Input: dimensioned drawing with shaded views. Units: mm. Origin: part minimum x, y, z. Coordinates: 2 decimals unless noted, no trailing zeros. Order: outer loops, then holes, each group sorted by start corner. A loop starts at its lowest first (then second) coordinate and runs counter-clockwise, first axis right, second up. Notation, with made-up numbers: (24, 1.5) - (74, 1.5) arc R13 ccw to (74, 6.5) - close; hole circle Ø9 at (6, 77). An arc over 180 degrees is marked (long way). Answer as CSV lines item,"result". Start each with the question number.
Item 1: Section D-D (x = 203.2). Output: boundary loops of the cut face in (y, z) (1 decimal).
Item 2: Section A-A (x = 164.5). Output: boundary loops of the cut face in (y, z) (1 decimal).
Item 3: Section C-C (y = 2.7). State how many separate pieces and enclosed holes the cut face has, and give its area (3 significant figures).
Item 4: First-contact query: pin 1 (3.5 mm diameter, centred on x = 12.7, z = 124.36, fed in from +Y); pin 2 (7.5 mm diameter, centred on x = 237.74, z = 124.36, fed in from +Y). Flat tips, straight axial feed; report the tip coordinate or a pass-through.
Item 5: Section B-B (z = 67.31). Output: boundary loops of the cut face in (x, y) (1 decimal).
Item 6: Material intervals for line 1 along X through (y, z) = (2.15, 124) (1 decimal); line 2 along Z through (x, y) = (165, 4.55) (1 decimal); line 3 along X through (y, z) = (2.3, 65) (1 decimal), sorted ascending.
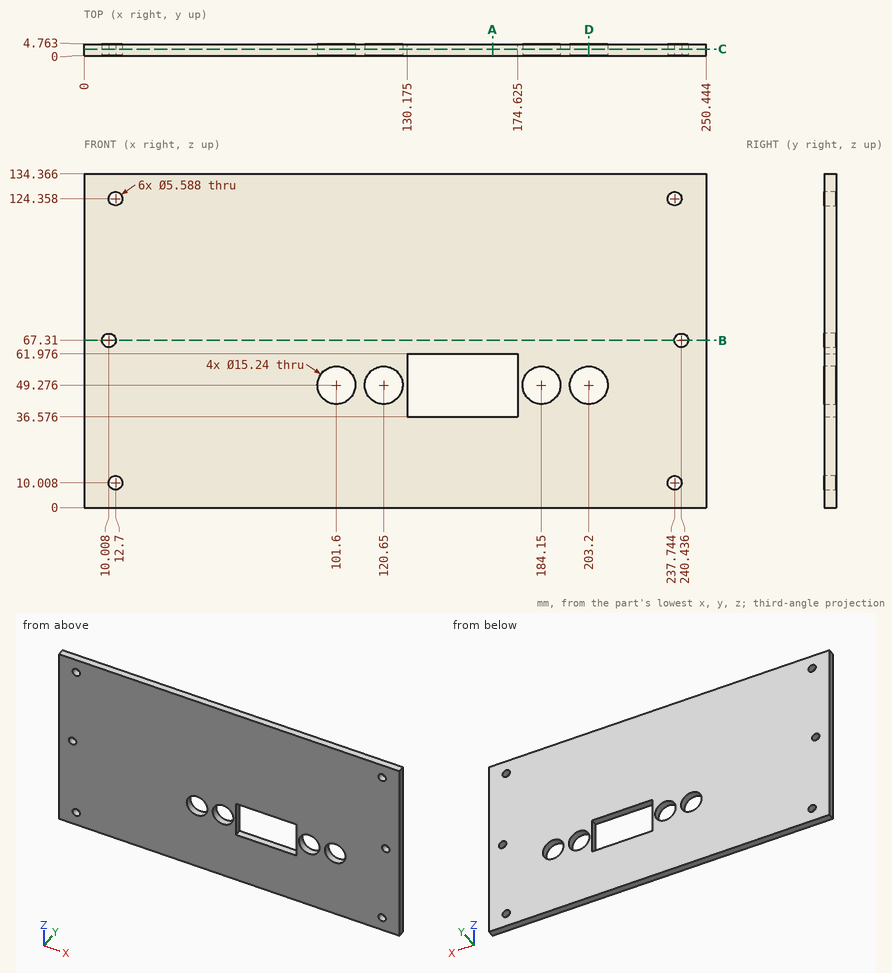
Determined:
1,outline,"(0, 0) - (4.8, 0) - (4.8, 41.7) - (0, 41.7) - close; (0, 56.9) - (4.8, 56.9) - (4.8, 134.4) - (0, 134.4) - close"
2,outline,"(0, 0) - (4.8, 0) - (4.8, 36.6) - (0, 36.6) - close; (0, 62) - (4.8, 62) - (4.8, 134.4) - (0, 134.4) - close"
3,separate pieces,"1"
3,enclosed holes,"11"
3,area,"31,600 mm^2"
4,pin 1,"passes through"
4,pin 2,"stops at y = 4.76"
5,outline,"(0, 0) - (7.2, 0) - (7.2, 4.8) - (0, 4.8) - close; (12.8, 0) - (237.6, 0) - (237.6, 4.8) - (12.8, 4.8) - close; (243.2, 0) - (250.4, 0) - (250.4, 4.8) - (243.2, 4.8) - close"
6,line 1,"x = 0 to 9.9, 15.5 to 235, 240.5 to 250.4"
6,line 2,"z = 0 to 36.6, 62 to 134.4"
6,line 3,"x = 0 to 8.4, 11.6 to 238.9, 242 to 250.4"
